Input: part model. Units: mm. Frame: model coordinates. Face numbers are marked on the shaded views. A direction names the side the tool comes from. Give positions to 0.01 mm unless a question says otherwise; leave off trailing zeros. Loops run counter-clockwise (first coordinate to the right, second up) from the corner with the lowest first, then second, coordinate; pieces in that order, holes last. Notation, with made-up numbers: M 89.25,-6.75 L 139.25,-6.75 A20 cw 139.25,16.25 Z; hole C -29.5,14.25 d4. An arc over 180 degrees is marked long. One line per item, written item: value. Start each with the question number.
(1) Access query for the marked faces 1, 2 and 3. Directions: +Z, -Z, +X, -X, +Y, -Y. A direction counts if a zero-diameter tool reaches every point of the face in a straight line with its end or side. Return the directions, or none.
(2) Ray query, line 1 along X through (y, z) = (-8, 1.9); line 2 along X through (y, z) = (0.75, 3.05); line 3 along X through (y, z) = (-0.75, 0.3). Return the intervals inside material, ascending. Write a range as from..to.
(3) Section C-C on y = -7.5. Output: boundary loops of the cut face in (x, z), plus the area to 3 significant figures.
(4) Section B-B on x = 0.5. Output: boundary loops of the cut face in (y, z), plus the area to 3 significant figures.
(5) Pull-direction query (X, two-part tool) for the marked faces 4, 5 and 6; classes: released by +X, released by -X, zero draft, split by the parting line, or undercut.
(6) Section D-D on x = -3. Output: boundary loops of the cut face in (y, z).
(7) Pin query (flat end, axial travel): P1, Ø1.5, axis at x = 6.5, y = 1, coming from the -Z side; P2, Ø1, axis at x = 3, z = 2, coming from the +Y side. Return the tip coordinate at first contact, or that it passes through.
(8) Section A-A on y = 7.5. Output: boundary loops of the cut face in (x, z).
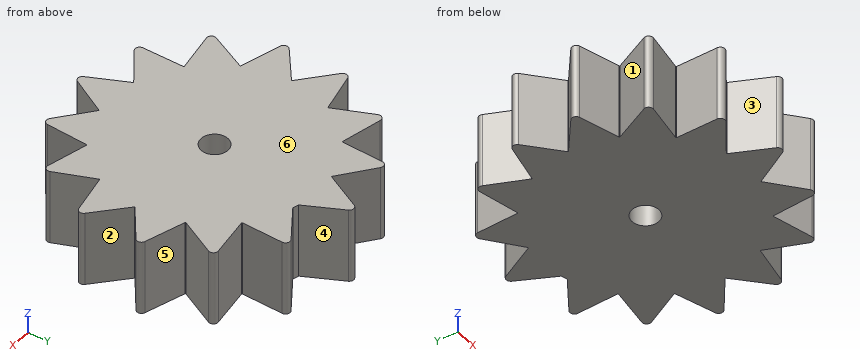
```python
from build123d import *

# Parameters (mm, degrees)
SKETCH1_R           = 7
SKETCH1_R_2         = 0.9
BOSS_EXTRUDE1_DEPTH = 5
BOSS_EXTRUDE2_START = -5
BOSS_EXTRUDE2_DEPTH = 5
CIRPATTERN1_COUNT   = 14
CIRPATTERN1_ANGLE   = 331.5


with BuildPart() as part:
    # Sketch1 → Boss-Extrude1 (new body)
    with BuildSketch(Plane.XY):
        Circle(SKETCH1_R)
        Circle(SKETCH1_R_2, mode=Mode.SUBTRACT)
    extrude(amount=BOSS_EXTRUDE1_DEPTH)

    # Sketch2 → Boss-Extrude2 (add)
    with BuildSketch(Plane.XY.offset(5).offset(BOSS_EXTRUDE2_START)):
        with BuildLine():
            ThreePointArc((0.267172205, 9.293419284), (0, 9.456967781), (-0.267172205, 9.293419284))
            Line((-0.267172205, 9.293419284), (-1.524265806, 6.832028524))
            ThreePointArc((-1.524265806, 6.832028524), (0, 7), (1.524265806, 6.832028524))
            Line((1.524265806, 6.832028524), (0.267172205, 9.293419284))
        make_face()
    boss_extrude2 = extrude(amount=BOSS_EXTRUDE2_DEPTH)

    # CirPattern1: Boss-Extrude2 ×14 about axis
    cirpattern1_axis = Axis((0, 0, 0), (0, 0, 1))
    for i in range(1, CIRPATTERN1_COUNT):
        add(boss_extrude2.rotate(cirpattern1_axis, i * CIRPATTERN1_ANGLE / (CIRPATTERN1_COUNT - 1)))


solid = part.part
```
Output values:
1. face 1: +Z, -Z, -X
1. face 2: +Z, -Z, +X
1. face 3: +Z, -Z, -Y
2. line 1: x = -4.46..-3.43, -1.12..0.73, 2.8..4.04
2. line 2: x = -7.74..-0.5, 0.5..8.3
2. line 3: x = -8.01..-0.5, 0.5..7.5
3. outline: M -4.46,0 L -2.74,0 L -2.74,5 L -4.46,5 Z; M -1.36,0 L 1,0 L 1,5 L -1.36,5 Z; M 2.18,0 L 4.07,0 L 4.07,5 L 2.18,5 Z
3. area: 29.9 mm²
4. outline: M -8.42,0 L -0.75,0 L -0.75,5 L -8.42,5 Z; M 0.75,0 L 8.84,0 L 8.84,5 L 0.75,5 Z
4. area: 78.8 mm²
5. face 4: undercut
5. face 5: released by +X
5. face 6: zero draft
6. outline: M -7.69,0 L 7.92,0 L 7.92,5 L -7.69,5 Z
7. P1: stops at z = 0
7. P2: stops at y = 7.81
8. outline: M -4.26,0 L -2.45,0 L -2.45,5 L -4.26,5 Z; M -1.18,0 L 1.18,0 L 1.18,5 L -1.18,5 Z; M 3.04,0 L 4.66,0 L 4.66,5 L 3.04,5 Z
